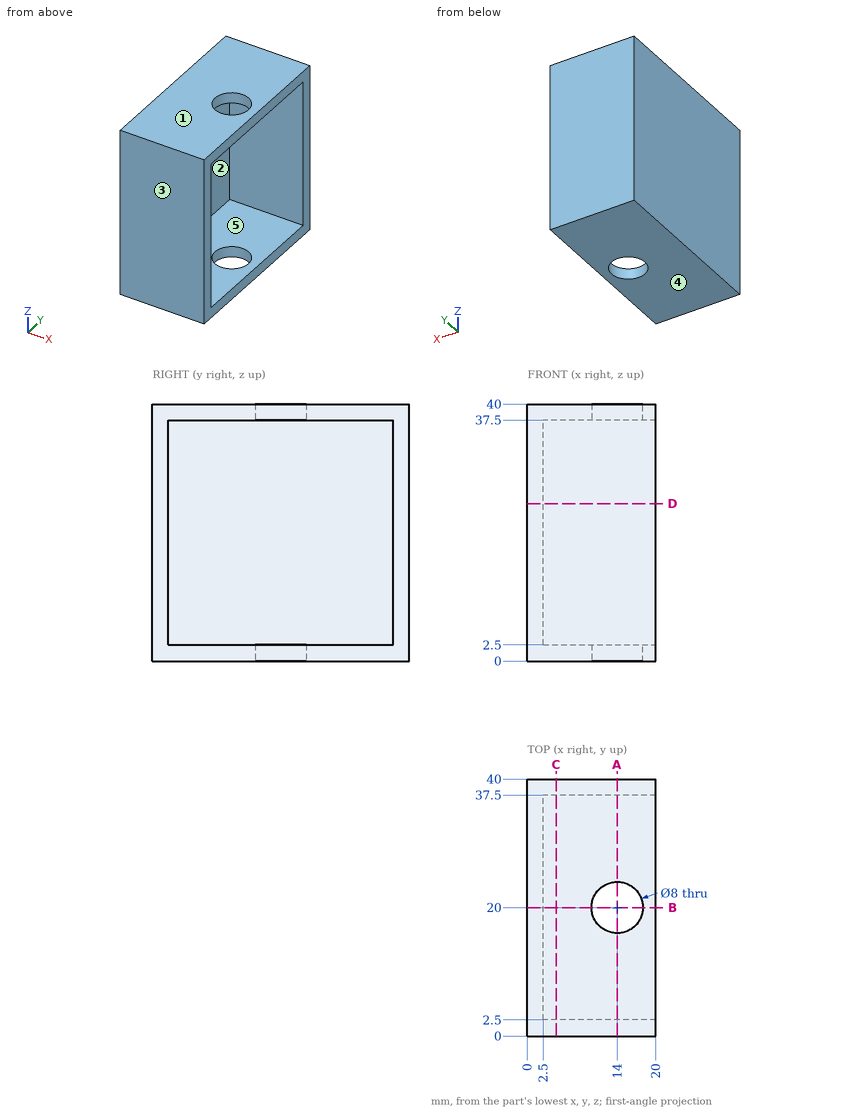
Check sheet for the drawn part. Datum: minimum x, y, z corner. Units: mm. A direction names the side the tool comes from. Give positions to 0.01 mm unless a question says otherwise; leave off trailing zeros. Order: outer loops, then holes, each group sorted by start corner. A loop starts at its lowest first (then second) coordinate and runs counter-clockwise, first axis right, second up.
1. Sectioned sample at A-A (x = 14). Record the boundary of the cut face in (y, z).
Completed:
outline: (0, 0) - (16, 0) - (16, 2.5) - (2.5, 2.5) - (2.5, 37.5) - (16, 37.5) - (16, 40) - (0, 40) - close; (24, 0) - (40, 0) - (40, 40) - (24, 40) - (24, 37.5) - (37.5, 37.5) - (37.5, 2.5) - (24, 2.5) - close
2. Draft check along Z on the marked faces 1, 2 and 3. Enter one of: pulls with the +Z half, pulls with the -Z half, needs draft (parallel to the pull), parting line crosses it, or undercut.
Completed:
face 1: pulls with the +Z half
face 2: undercut
face 3: needs draft
3. Sectioned sample at D-D (z = 24.5). Record the boundary of the cut face in (x, y), then the cut area to 4 significant figures.
Completed:
outline: (0, 0) - (20, 0) - (20, 2.5) - (2.5, 2.5) - (2.5, 37.5) - (20, 37.5) - (20, 40) - (0, 40) - close
area: 187.5 mm2
4. Sectioned sample at C-C (x = 4.5). Record the boundary of the cut face in (y, z), then the cut area to 3 significant figures.
Completed:
outline: (0, 0) - (40, 0) - (40, 40) - (0, 40) - close; hole (2.5, 2.5) - (37.5, 2.5) - (37.5, 37.5) - (2.5, 37.5) - close
area: 375 mm2
5. Depth check by flat-ended pin: pin 1 (5 mm diameter, centred on x = 14.5, z = 27, fed in from -Y); pin 2 (17.5 mm diameter, centred on y = 18, z = 12.5, fed in from +X). Enter the tip coordinate at first touch or a pass-through.
Completed:
pin 1: stops at y = 0
pin 2: stops at x = 2.5
6. Access from +Z, -Z, +X, -X, +Y, -Y to the whole of each face (thin tool, end or side, straight path). Record for the marked faces 4 and 5.
Completed:
face 4: -Z, +X, -X, +Y, -Y
face 5: +X
7. Scan lines: line 1 (Y direction, x = 14, z = 19.5); line 2 (X direction, y = 20, z = 38.35). Record each from-to range of solid material in increasing order.
Completed:
line 1: y = 0 to 2.5, 37.5 to 40
line 2: x = 0 to 10, 18 to 20
8. Sectioned sample at B-B (y = 20). Record the boundary of the cut face in (x, z), then the cut area to 4 significant figures.
Completed:
outline: (0, 0) - (10, 0) - (10, 2.5) - (2.5, 2.5) - (2.5, 37.5) - (10, 37.5) - (10, 40) - (0, 40) - close; (18, 0) - (20, 0) - (20, 2.5) - (18, 2.5) - close; (18, 37.5) - (20, 37.5) - (20, 40) - (18, 40) - close
area: 147.5 mm2
